Here's how the part is built. I have some questions about the finished solid (model axes, mm). A direction names the side the tool comes from. Coordinates: 2 decimals unless noted, no trailing zeros. Order: outer loops, then holes, each group sorted by start corner. A loop starts at its lowest first (then second) coordinate and runs counter-clockwise, first axis right, second up.
```python
from build123d import *

# Parameters (mm, degrees)
SKETCH1_W           = 6.35
SKETCH1_H           = 25.4
EXTRUDE_THIN1_DEPTH = 5.08
FILLET4_R           = 1.27
FILLET5_R           = 1.27
FILLET6_R           = 1.27
SKETCH5_R           = 1.651
CUT_EXTRUDE1_DEPTH  = 6.35
SKETCH8_R           = 3.81
BOSS_EXTRUDE1_DEPTH = 6.35
SKETCH12_R          = 2.3999952
BOSS_EXTRUDE2_DEPTH = 19.05
LPATTERN1_COUNT     = 2
LPATTERN1_PITCH     = 18.034


with BuildPart() as part:
    # Sketch1 → Extrude-Thin1 (new body)
    with BuildSketch(Plane(origin=(0, 0, 0), x_dir=(1, 0, 0), z_dir=(0, 1, 0))):
        with Locations((-0.347720453, -19.952908818)):
            Rectangle(SKETCH1_W, SKETCH1_H)
    extrude(amount=EXTRUDE_THIN1_DEPTH)

    # Fillet4
    fillet4_edges = [part.edges().sort_by_distance(p)[0] for p in [
        (-3.522720453, 2.54, 32.652908818),
    ]]
    fillet(fillet4_edges, radius=FILLET4_R)

    # Fillet5
    fillet5_edges = [part.edges().sort_by_distance(p)[0] for p in [
        (2.827279547, 2.54, 32.652908818),
    ]]
    fillet(fillet5_edges, radius=FILLET5_R)

    # Fillet6
    fillet6_edges = [part.edges().sort_by_distance(p)[0] for p in [
        (-3.522720453, 2.54, 7.252908818),
        (2.827279547, 2.54, 7.252908818),
    ]]
    fillet(fillet6_edges, radius=FILLET6_R)

    # Sketch5 → Cut-Extrude1 (cut)
    with BuildSketch(Plane(origin=(0, 5.08, 0), x_dir=(1, 0, 0), z_dir=(0, 1, 0))):
        with Locations((-0.381, -29.972)):
            Circle(SKETCH5_R)
    cut_extrude1 = extrude(amount=-CUT_EXTRUDE1_DEPTH, mode=Mode.SUBTRACT)

    # Sketch8 → Boss-Extrude1 (add)
    with BuildSketch(Plane(origin=(2.827279547, 0, 0), x_dir=(0, 0, -1), z_dir=(1, 0, 0))):
        with Locations((-12.042526448, 3.1242)):
            Circle(SKETCH8_R)
    extrude(amount=BOSS_EXTRUDE1_DEPTH)

    # Sketch12 → Boss-Extrude2 (add)
    with BuildSketch(Plane(origin=(2.827279547, 0, 0), x_dir=(0, 0, -1), z_dir=(1, 0, 0))):
        with Locations((-12.042526448, 3.1242)):
            Circle(SKETCH12_R)
    extrude(amount=BOSS_EXTRUDE2_DEPTH)

    # LPattern1: Cut-Extrude1 ×2
    with Locations(*[(0, 0, -i * LPATTERN1_PITCH) for i in range(1, LPATTERN1_COUNT)]):
        add(cut_extrude1, mode=Mode.SUBTRACT)


solid = part.part
```
Q1. If we section it at C-C on z = 26.5: Write out the boundary of the cut face in (x, y).
Q2. If we section it at B-B on z = 29.25: Write out the boundary of the cut face in (x, y).
Q3. Will these pins go through, and if not, where does the flat tip stop? pin 1 (1.9 mm diameter, centred on x = -1.5, z = 22, fed in from -Y); pin 2 (8 mm diameter, centred on x = 15, z = 18, fed in from -Y); pin 3 (1.9 mm diameter, centred on x = 0.5, z = 19, fed in from +Y).
Q4. If we section it at A-A on x = -1.5: Write out the boundary of the cut face in (y, z).
Q5. I need wall thicknesses on L1, parallel to Z at x = 20, y = 3.25; L2, parallel to Z at x = 0, y = 1; L3, parallel to X at y = 2.25, z = 29.5. Which ranges of each line are inside material? Lowest first, please.
Q6. For faces 1 (the flat face through (0, 3, 7.253)), 2 (the flat face through (2.827, 6, 12)), 3 (the flat face through (2.827, 0.5, 8.9)), 4 (the flat face through (0, 0, 20)), 5 (the cylindrical face through (15.438, 1.664, 13.947)), which set-ups out of +Z, -Z, +X, -X, +Y, -Y let a thin tool reach every point of the face, with its end or its side?
Q7. If we section it at D-D on z = 12.25: Write out the boundary of the cut face in (x, y).
Reply:
1. outline: (-3.52, 0) - (2.83, 0) - (2.83, 5.08) - (-3.52, 5.08) - close
2. outline: (-3.52, 0) - (-1.87, 0) - (-1.87, 5.08) - (-3.52, 5.08) - close; (1.1, 0) - (2.83, 0) - (2.83, 5.08) - (1.1, 5.08) - close
3. pin 1: stops at y = 0
3. pin 2: stops at y = 1.74
3. pin 3: stops at y = 5.08
4. outline: (0, 7.25) - (5.08, 7.25) - (5.08, 10.72) - (0, 10.72) - close; (0, 13.15) - (5.08, 13.15) - (5.08, 28.76) - (0, 28.76) - close; (0, 31.19) - (5.08, 31.19) - (5.08, 32.65) - (0, 32.65) - close
5. L1: z = 9.65 to 14.44
5. L2: z = 7.25 to 10.33, 13.54 to 28.37, 31.58 to 32.65
5. L3: x = -3.52 to -1.96, 1.2 to 2.83
6. face 1: -Z, +X, -X, +Y, -Y
6. face 2: +Z, -Z, -X, +Y
6. face 3: -Z, +X, -Y
6. face 4: +Z, -Z, -X, -Y
6. face 5: +X
7. outline: (-3.52, 0) - (-2, 0) - (-2, 5.08) - (-3.52, 5.08) - close; (1.24, 0) - (2.83, 0) - (2.83, -0.68) - (9.18, -0.68) - (9.18, 0.73) - (21.88, 0.73) - (21.88, 5.52) - (9.18, 5.52) - (9.18, 6.93) - (2.83, 6.93) - (2.83, 5.08) - (1.24, 5.08) - close
